Can you work these out from the model? Positions are in its coordinate system, mm. A direction names the side the tool comes from. Round coordinates to 2 decimals unless told otherwise and drop trailing zeros. Order: outer loops, then holes, each group sorted by start corner. A loop starts at its lowest first (then second) coordinate and runs counter-clockwise, first axis right, second up. Notation, with made-up numbers: M 88.5,29.25 L 119.5,29.25 A13 ccw 119.5,53.25 Z; hole C 80,82.25 d3. An arc over 180 degrees is marked long. One line per question, with ' | ' between items.
```python
from build123d import *

# Parameters (mm, degrees)
BOSS_EXTRUDE1_DEPTH = 340.5
FILLET1_R           = 1


with BuildPart() as part:
    # Sketch1 → Boss-Extrude1 (new body)
    with BuildSketch(Plane.XY):
        Polygon((0, 0), (-8.5, 0), (-8.5, 8.5), (-6.5, 8.5), (-6.5, 2), (0, 2), align=None)
    extrude(amount=BOSS_EXTRUDE1_DEPTH)

    # Fillet1
    fillet1_edges = [part.edges().sort_by_distance(p)[0] for p in [
        (-8.5, 0, 170.25),
    ]]
    fillet(fillet1_edges, radius=FILLET1_R)

    # Sketch7 → CSK for M3 Countersunk Flat Head Screw1 (revolve, cut)
    with BuildSketch(Plane(origin=(-8.5, 4.5, 21), x_dir=(0, 0, 1), z_dir=(0, 1, 0))):
        Polygon((0, 0), (0, 10.521463052), (1.7, 9.5), (1.7, 1.75), (3.15, 0.3), (3.15, 0), align=None)
    revolve(axis=Axis((-14.85, 4.5, 21), (1, 0, 0)), mode=Mode.SUBTRACT)

    # Sketch7 at point 2 (carried to point 2, square into its face) → CSK for M3 Countersunk Flat Head Scr 2 (revolve, cut)
    with BuildSketch(Plane(origin=(-4, 0, 65.25), x_dir=(0, 0, 1), z_dir=(-1, 0, 0))):
        Polygon((0, 0), (0, 10.521463052), (1.7, 9.5), (1.7, 1.75), (3.15, 0.3), (3.15, 0), align=None)
    revolve(axis=Axis((-4, -6.35, 65.25), (0, 1, 0)), mode=Mode.SUBTRACT)

    # Sketch7 at point 3 (carried to point 3, square into its face) → CSK for M3 Countersunk Flat Head Scr 3 (revolve, cut)
    with BuildSketch(Plane(origin=(-4, 0, 143.19999924), x_dir=(0, 0, 1), z_dir=(-1, 0, 0))):
        Polygon((0, 0), (0, 10.521463052), (1.7, 9.5), (1.7, 1.75), (3.15, 0.3), (3.15, 0), align=None)
    revolve(axis=Axis((-4, -6.35, 143.19999924), (0, 1, 0)), mode=Mode.SUBTRACT)

    # Sketch7 at point 4 (carried to point 4, square into its face) → CSK for M3 Countersunk Flat Head Scr 4 (revolve, cut)
    with BuildSketch(Plane(origin=(-4, 0, 275.25), x_dir=(0, 0, 1), z_dir=(-1, 0, 0))):
        Polygon((0, 0), (0, 10.521463052), (1.7, 9.5), (1.7, 1.75), (3.15, 0.3), (3.15, 0), align=None)
    revolve(axis=Axis((-4, -6.35, 275.25), (0, 1, 0)), mode=Mode.SUBTRACT)

    # Sketch7 at point 5 (carried to point 5, square into its face) → CSK for M3 Countersunk Flat Head Scr 5 (revolve, cut)
    with BuildSketch(Plane(origin=(-8.5, 4.5, 330.5), x_dir=(0, 0, 1), z_dir=(0, 1, 0))):
        Polygon((0, 0), (0, 10.521463052), (1.7, 9.5), (1.7, 1.75), (3.15, 0.3), (3.15, 0), align=None)
    revolve(axis=Axis((-14.85, 4.5, 330.5), (1, 0, 0)), mode=Mode.SUBTRACT)


solid = part.part
```
(1) If we section it at A-A on y = 4.5: Please give me the cut outline in (x, z).
Final values:
outline: M -8.5,0 L -6.5,0 L -6.5,19.3 L -6.75,19.3 L -8.2,17.85 L -8.5,17.85 Z; M -8.5,24.15 L -8.2,24.15 L -6.75,22.7 L -6.5,22.7 L -6.5,328.8 L -6.75,328.8 L -8.2,327.35 L -8.5,327.35 Z; M -8.5,333.65 L -8.2,333.65 L -6.75,332.2 L -6.5,332.2 L -6.5,340.5 L -8.5,340.5 Z
(2) If we section it at B-B on x = -4: Please give me the cut outline in (y, z).
Final values:
outline: M 0,0 L 2,0 L 2,63.55 L 1.75,63.55 L 0.3,62.1 L 0,62.1 Z; M 0,68.4 L 0.3,68.4 L 1.75,66.95 L 2,66.95 L 2,141.5 L 1.75,141.5 L 0.3,140.05 L 0,140.05 Z; M 0,146.35 L 0.3,146.35 L 1.75,144.9 L 2,144.9 L 2,273.55 L 1.75,273.55 L 0.3,272.1 L 0,272.1 Z; M 0,278.4 L 0.3,278.4 L 1.75,276.95 L 2,276.95 L 2,340.5 L 0,340.5 Z
(3) Will these pins go through, and if not, where does the flat tip stop? pin 1 Ø2 at (x, z) = (-4, 65.25) entering from -Y; pin 2 Ø4.5 at (x, z) = (-4, 143.2) entering from +Y; pin 3 Ø4 at (y, z) = (4.5, 330.5) entering from +X.
Final values:
pin 1: through | pin 2: y = 2 | pin 3: x = -6.5
(4) Thinking about a two-plate mould opening in Z: for faces 1 (the flat face through (-6, 1, 0)), 2 (the cylindrical face through (-8.35, 2.37, 18.68)), 3 (the flat face through (-3, 2, 168)), which applies, released by +Z, released by -Z, zero draft, split by the parting line, or undercut?
Final values:
face 1: released by -Z | face 2: undercut | face 3: zero draft
(5) On a 3-axis mill with a long thin cutter (end or side, diameter ignored), from which of +Z, -Z, +X, -X, +Y, -Y can I reach the whole of each face in a straight line? I mean faces 4 (the cylindrical face through (-8.35, 5.71, 333.41)), 5 (the flat face through (-6.5, 5, 168)), 6 (the cylindrical face through (-1.87, 0.15, 62.93)). Say none if no direction works.
Final values:
face 4: -X | face 5: +Z, -Z, +X, +Y | face 6: -Y
(6) Please list where these lines run through material, in increasing order: probe 1 along Z at (x, y) = (-4, 1.8); probe 2 along Z at (x, y) = (-8.35, 4.5); probe 3 along X at (y, z) = (1.8, 275.25). Write a range as [from, to].
Final values:
probe 1: [0, 63.55], [66.95, 141.5], [144.9, 273.55], [276.95, 340.5] | probe 2: [0, 17.85], [24.15, 327.35], [333.65, 340.5] | probe 3: [-8.5, -5.7], [-2.3, 0]
(7) If we section it at C-C on z = 109: Please give me the cut outline in (x, y).
Final values:
outline: M -8.5,1 A1 ccw -7.5,0 L 0,0 L 0,2 L -6.5,2 L -6.5,8.5 L -8.5,8.5 Z
